For this review, take the finished solid that the model builds, in its own axes (mm). A direction names the side the tool comes from. Round coordinates to 2 decimals unless told otherwise and drop trailing zeros. Order: outer loops, then holes, each group sorted by start corner. A loop starts at its lowest first (then second) coordinate and runs counter-clockwise, first axis right, second up. Notation, with made-up numbers: (57, 20.25) - (75, 20.25) arc R25 cw to (75, 59.25) - close; hole circle Ø4 at (88.5, 3.25). An arc over 180 degrees is marked (long way). One line per question, with ' | ' between items.
```python
from build123d import *

# Parameters (mm, degrees)
BOSS_EXTRUDE1_DEPTH = 35
SKETCH2_R           = 2
CUT_EXTRUDE1_DEPTH  = 50
SKETCH3_R           = 1.5
SKETCH3_R_2         = 1
CUT_EXTRUDE2_DEPTH  = 50


with BuildPart() as part:
    # Sketch1 → Boss-Extrude1 (new body)
    with BuildSketch(Plane.XY):
        Polygon((0, 50), (0, 0), (50, 0), (50, 3), (3, 3), (3, 50), align=None)
    extrude(amount=BOSS_EXTRUDE1_DEPTH)

    # Sketch2 → Cut-Extrude1 (cut)
    with BuildSketch(Plane(origin=(0, 3, 0), x_dir=(1, 0, 0), z_dir=(0, 1, 0))):
        with Locations(Location((19, -11.5, 0), (0, 0, 270))):
            Circle(SKETCH2_R)
        with Locations(Location((34, -11.5, 0), (0, 0, 270))):
            Circle(SKETCH2_R)
        with Locations(Location((34, -23.5, 0), (0, 0, 270))):
            Circle(SKETCH2_R)
        with Locations(Location((19, -23.5, 0), (0, 0, 270))):
            Circle(SKETCH2_R)
    extrude(amount=-CUT_EXTRUDE1_DEPTH, mode=Mode.SUBTRACT)

    # Sketch3 → Cut-Extrude2 (cut)
    with BuildSketch(Plane(origin=(3, 0, 0), x_dir=(0, 0, -1), z_dir=(1, 0, 0))):
        with Locations((-17.5, 26.5)):
            Circle(SKETCH3_R)
        with Locations((-13.020503905, 20.484676672)):
            Circle(SKETCH3_R_2)
        with Locations((-21.979496095, 32.515323328)):
            Circle(SKETCH3_R_2)
        with Locations((-23.771294533, 34.921452659)):
            Circle(SKETCH3_R_2)
        with Locations((-25.563092971, 37.32758199)):
            Circle(SKETCH3_R_2)
        with Locations((-27.354891409, 39.733711321)):
            Circle(SKETCH3_R_2)
        with Locations((-11.228705467, 18.078547341)):
            Circle(SKETCH3_R_2)
        with Locations((-9.436907029, 15.67241801)):
            Circle(SKETCH3_R_2)
        with Locations((-7.645108591, 13.266288679)):
            Circle(SKETCH3_R_2)
    extrude(amount=-CUT_EXTRUDE2_DEPTH, mode=Mode.SUBTRACT)


solid = part.part
```
(1) Mouldability with a two-part tool opening along Z and no side actions: class faces 3 (the cylindrical face through (20.983, 1.521, 23.24)), 4 (the cylindrical face through (1.521, 14.696, 9.654)), 5 (the flat face through (2.7, 14, 35)), 6 (the flat face through (2, 50, 17)) as released by +Z, released by -Z, zero draft, split by the parting line, or undercut.
Output values:
face 3: undercut | face 4: undercut | face 5: released by +Z | face 6: zero draft
(2) For probe 1 along X at (y, z) = (1.35, 11.5); probe 2 along Y at (x, z) = (45.5, 6.5), list the stretches that pass through material, from the lowest coordinate up. Write a range as [from, to].
Output values:
probe 1: [0, 17], [21, 32], [36, 50] | probe 2: [0, 3]
(3) Insertion check: pin 1 (1.2 mm diameter, centred on y = 13.27, z = 7.65, fed in from +X); pin 2 (5 mm diameter, centred on x = 8, z = 30.5, fed in from +Y); pin 3 (4 mm diameter, centred on y = 34.5, z = 12, fed in from +X). Each pin has a flat end and moves straight along its axis. Give the tip position at first contact, or say it passes through.
Output values:
pin 1: through | pin 2: y = 3 | pin 3: x = 3
(4) We need section A-A on y = 26.5. State the section outline as (x, z) points, plus the area to 3 significant figures.
Output values:
outline: (0, 0) - (3, 0) - (3, 16) - (0, 16) - close; (0, 19) - (3, 19) - (3, 35) - (0, 35) - close | area: 96.0 mm^2
(5) For faces 1 (the cylindrical face through (1.5, 12.3, 7.9)), 2 (the flat face through (27, 3, 17)), list the 3-axis set-ups (+Z, -Z, +X, -X, +Y, -Y) from which the entire face can be reached by the end or side of a thin tool; tool diameter is ignored.
Output values:
face 1: +X, -X | face 2: +Z, -Z, +X, +Y
(6) We need section B-B on z = 17.5. State the section outline as (x, y) points.
Output values:
outline: (0, 0) - (50, 0) - (50, 3) - (3, 3) - (3, 25) - (0, 25) - close; (0, 28) - (3, 28) - (3, 50) - (0, 50) - close
(7) We need section C-C on x = 39. State the section outline as (y, z) points, plus the area to 3 significant figures.
Output values:
outline: (0, 0) - (3, 0) - (3, 35) - (0, 35) - close | area: 105 mm^2
(8) We need section D-D on z = 32.5. State the section outline as (x, y) points, plus the area to 3 significant figures.
Output values:
outline: (0, 0) - (50, 0) - (50, 3) - (3, 3) - (3, 50) - (0, 50) - close | area: 291 mm^2
